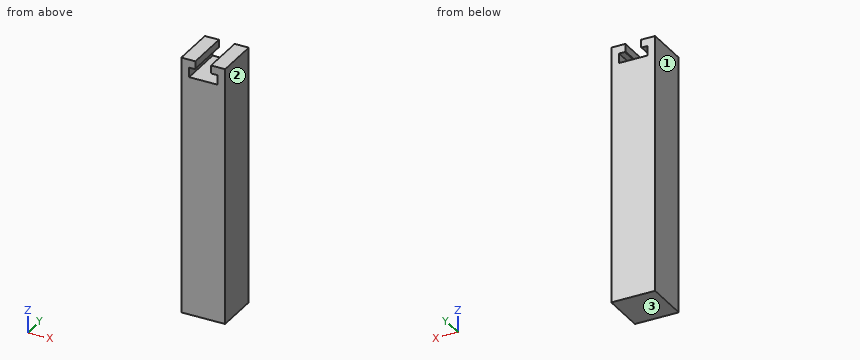
from build123d import *

# Parameters (mm, degrees)
F0_W     = 9.9568
F0_H     = 58.5216
F1_DEPTH = 9.9568
F3_DEPTH = 9.9578
F4_SIZE  = 0.127


with BuildPart() as f1:
    # F0 (on Front) → F1 (new body)
    with BuildSketch(Plane.XZ):
        with Locations((4.9784, -29.2608)):
            Rectangle(F0_W, F0_H)
    extrude(amount=-F1_DEPTH)

    # F2 (on face) → F3 (cut, through all)
    with BuildSketch(Plane.XZ):
        Polygon((6.7564, 1.562734), (3.2004, 1.562903), (3.2004, -1.8288), (1.778, -1.8288), (1.778, -4.0132), (8.1788, -4.0132), (8.1788, -1.8288), (6.7564, -1.8288), align=None)
    extrude(amount=-F3_DEPTH, mode=Mode.SUBTRACT)

    # F4
    f4_edges = [f1.edges().sort_by_distance(p)[0] for p in [
        (3.2004, 4.9784, -1.8288),
        (6.7564, 4.9784, -1.8288),
    ]]
    chamfer(f4_edges, length=F4_SIZE)


solid = f1.part
Can you work these out from the model? Positions are in its coordinate system, mm. Face numbers are marked on the shaded views. Give positions to 0.01 mm unless a question says otherwise; leave off trailing zeros. Loops run counter-clockwise (first coordinate to the right, second up) from the corner with the lowest first, then second, coordinate; pieces in that order, holes last. Notation, with made-up numbers: (72.5, -27.75) - (116.5, -27.75) arc R28 ccw to (116.5, -9.75) - close; hole circle Ø8 at (-2, 1.25). An arc over 180 degrees is marked (long way). Return JSON: item names as keys, results as strings.
1. We'd pull the mould along X, two halves only. Please class the marked faces 1, 2 and 3: +X half, -X half, draft (parallel to the pull), parting line (faces both ways), or undercut.
Output values:
{"face 1": "-X half", "face 2": "+X half", "face 3": "draft"}
2. If I drill on line 1 (Z direction, x = 2.75, y = 7); line 2 (X direction, y = 2, z = -2.5); line 3 (Z direction, x = 3.75, y = 5.5), over which ranges is the centre line in solid material (lowest first)?
Output values:
{"line 1": "z = -58.52 to -4.01, -1.83 to 0", "line 2": "x = 0 to 1.78, 8.18 to 9.96", "line 3": "z = -58.52 to -4.01"}
3. I want a section at B-B on y = 9.25. Please give me the cut outline in (x, z).
Output values:
{"outline": "(0, -58.52) - (9.96, -58.52) - (9.96, 0) - (6.76, 0) - (6.76, -1.7) - (6.88, -1.83) - (8.18, -1.83) - (8.18, -4.01) - (1.78, -4.01) - (1.78, -1.83) - (3.07, -1.83) - (3.2, -1.7) - (3.2, 0) - (0, 0) - close"}
4. I want a section at A-A on x = 2.5. Please give me the cut outline in (y, z).
Output values:
{"outline": "(0, -58.52) - (9.96, -58.52) - (9.96, -4.01) - (0, -4.01) - close; (0, -1.83) - (9.96, -1.83) - (9.96, 0) - (0, 0) - close"}
